Work out the finished part from the listing and answer in its coordinate system (mm). Face numbers are marked on the shaded views. A direction names the side the tool comes from. Round coordinates to 2 decimals unless told otherwise and drop trailing zeros. Order: outer loops, then holes, each group sorted by start corner. A loop starts at its lowest first (then second) coordinate and runs counter-clockwise, first axis right, second up. Notation, with made-up numbers: (72, 34) - (80, 34) arc R34 cw to (80, 64) - close; hole circle Ø6 at (62, 71). An arc over 180 degrees is marked (long way). Put each result on its own line as item: value.
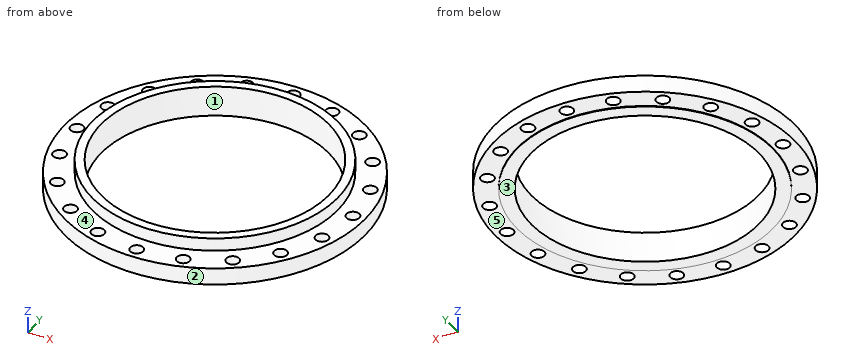
```python
from build123d import *

# Parameters (mm, degrees)
SKETCH2_R               = 16
BOSS_EXTRUDE1_DEPTH     = 1.81
SKETCH3_R               = 13.06
BOSS_EXTRUDE2_DEPTH     = 3.19
SKETCH4_R               = 13.625
BOSS_EXTRUDE3_DEPTH     = 0.0625
SKETCH5_R               = 12.125
CUT_EXTRUDE1_DEPTH      = 56
CUT_EXTRUDE1_DEPTH_BACK = 4.0625
SKETCH6_R               = 0.69
CUT_EXTRUDE2_DEPTH      = 2.0625
CIRPATTERN1_COUNT       = 20
SCALE1_SCALE            = 25.4


with BuildPart() as part:
    # Sketch2 → Boss-Extrude1 (new body)
    with BuildSketch(Plane.XY):
        Circle(SKETCH2_R)
    extrude(amount=BOSS_EXTRUDE1_DEPTH)

    # Sketch3 → Boss-Extrude2 (add)
    with BuildSketch(Plane.XY):
        Circle(SKETCH3_R)
    extrude(amount=BOSS_EXTRUDE2_DEPTH)

    # Sketch4 → Boss-Extrude3 (add)
    with BuildSketch(Plane.XY):
        Circle(SKETCH4_R)
    extrude(amount=-BOSS_EXTRUDE3_DEPTH)

    # Sketch5 → Cut-Extrude1 (cut, two sides)
    with BuildSketch(Plane.XY) as cut_extrude1_sk:
        Circle(SKETCH5_R)
    extrude(amount=CUT_EXTRUDE1_DEPTH, mode=Mode.SUBTRACT)
    extrude(cut_extrude1_sk.sketch, amount=-CUT_EXTRUDE1_DEPTH_BACK, mode=Mode.SUBTRACT)

    # Sketch6 → Cut-Extrude2 (cut)
    with BuildSketch(Plane.XY):
        with Locations((0, 14.75)):
            Circle(SKETCH6_R)
    cut_extrude2 = extrude(amount=CUT_EXTRUDE2_DEPTH, mode=Mode.SUBTRACT)

    # CirPattern1: Cut-Extrude2 ×20 about axis
    cirpattern1_axis = Axis((0, 0, 0), (0, 0, 1))
    for i in range(1, CIRPATTERN1_COUNT):
        add(cut_extrude2.rotate(cirpattern1_axis, i * 360 / CIRPATTERN1_COUNT), mode=Mode.SUBTRACT)


with BuildPart() as part_1:
    # Scale1: scaled about (0, 0, 1.135631503)
    add(part.part.scale(SCALE1_SCALE).moved(Location((0, 0, -27.709408673))))


solid = part_1.part
```
1) Given pin 1 Ø12 at (x, z) = (-312, -20) entering from +Y; pin 2 Ø3 at (y, z) = (56.5, -12) entering from +X; pin 3 Ø21 at (x, y) = (303.1, 220.21) entering from +Z; pin 4 Ø4 at (y, z) = (213, -15) entering from -X, each flat-ended and moving along its own axis, determine where each tip first touches the part or whether it passes through.
Findings below:
pin 1: stops at y = 267.44
pin 2: stops at x = 402.66
pin 3: passes through
pin 4: stops at x = -347.33
2) Straight lines are drawn through the part: L1, parallel to Y at x = 235.5, z = -19; L2, parallel to Y at x = 107, z = 9; L3, parallel to X at y = 111, z = -12. For each, find the intervals that lie inside material, in ascending order. Write a range as from..to.
Findings below:
L1: y = -331.21..-311.67, -294.53..-198.46, 198.46..294.53, 311.67..331.21
L2: y = -392.06..-371.49, -341.14..-288.79, 288.79..341.14, 371.49..392.06
L3: x = -390.95..-373.18, -339.45..-287.28, 287.28..339.45, 373.18..390.95
3) For the marked faces 4 and 5, determine the directions among +Z, -Z, +X, -X, +Y, -Y from which every point of the face is accessible in a straight line to the end or side of a thin tool.
Findings below:
face 4: +Z
face 5: -Z
4) A cutting plane is placed at A-A on x = 0. Write down the section's boundary in (y, z) (3 decimals), then the cut area to 3 significant figures.
Findings below:
outline: (-406.4, -27.709) - (-392.176, -27.709) - (-392.176, 18.265) - (-406.4, 18.265) - close; (-357.124, -27.709) - (-346.075, -27.709) - (-346.075, -29.297) - (-307.975, -29.297) - (-307.975, 53.317) - (-331.724, 53.317) - (-331.724, 18.265) - (-357.124, 18.265) - close; (307.975, -29.297) - (346.075, -29.297) - (346.075, -27.709) - (357.124, -27.709) - (357.124, 18.265) - (331.724, 18.265) - (331.724, 53.317) - (307.975, 53.317) - close; (392.176, -27.709) - (406.4, -27.709) - (406.4, 18.265) - (392.176, 18.265) - close
area: 7,610 mm2
5) A cutting plane is placed at D-D on y = 55.5. Write down the section's boundary in (x, z).
Findings below:
outline: (-402.59, -27.71) - (-341.6, -27.71) - (-341.6, -29.3) - (-302.93, -29.3) - (-302.93, 53.32) - (-327.05, 53.32) - (-327.05, 18.26) - (-402.59, 18.26) - close; (302.93, -29.3) - (341.6, -29.3) - (341.6, -27.71) - (402.59, -27.71) - (402.59, 18.26) - (327.05, 18.26) - (327.05, 53.32) - (302.93, 53.32) - close
6) For a pull along X with two mould halves and no side action, classify the marked faces 1, 2 and 3 as pulls with the +X half, pulls with the -X half, needs draft (parallel to the pull), parting line crosses it, or undercut.
Findings below:
face 1: undercut
face 2: parting line crosses it
face 3: needs draft
7) A cutting plane is placed at B-B on y = -45. Write down the section's boundary in (x, z).
Findings below:
outline: (-403.9, -27.71) - (-343.14, -27.71) - (-343.14, -29.3) - (-304.67, -29.3) - (-304.67, 53.32) - (-328.66, 53.32) - (-328.66, 18.26) - (-403.9, 18.26) - close; (304.67, -29.3) - (343.14, -29.3) - (343.14, -27.71) - (403.9, -27.71) - (403.9, 18.26) - (328.66, 18.26) - (328.66, 53.32) - (304.67, 53.32) - close
8) A cutting plane is placed at C-C on z = -10. Give the number of separate pieces and of enclosed holes in the cut face, then the cut area to 3 significant figures.
Findings below:
separate pieces: 1
enclosed holes: 21
area: 202,000 mm2
